Model file for the job. Use its own axes, mm. A direction names the side the tool comes from. Round coordinates to 2 decimals unless told otherwise and drop trailing zeros. Loops run counter-clockwise (first coordinate to the right, second up) from the corner with the lowest first, then second, coordinate; pieces in that order, holes last. Notation, with made-up numbers: (29.25, 12.5) -> (36.25, 12.5) arc R22 cw to (36.25, 35.5) -> close; hole circle Ø10 at (-21, 83.5). An arc over 180 degrees is marked (long way). Use a Markdown table: item, result. Add a question column.
```python
from build123d import *

# Parameters (mm, degrees)
BODY_START           = -10
BODY_DEPTH           = 20
M3_CLEARANCE_HOLE1_D = 3.4
CUT_EXTRUDE1_REACH   = 34.243
SKETCH4_R            = 2.5


# Read off the part's stored shape, not the designer's step: Body
with BuildPart() as part:
    # Body outline → Body (new body)
    with BuildSketch(Plane.XY.offset(BODY_START)):
        Polygon((9.25, 24.25), (9.25, 4.25), (-1.25, 4.25), (-1.25, 24.25), (-5.75, 24.25), (-5.75, 4.25), (-13, 4.25), (-13, -1.25), (13, -1.25), (13, 24.25), align=None)
    extrude(amount=BODY_DEPTH)

    # M3 Clearance Hole1 (through all)
    with Locations(Plane(origin=(0, -1.25, 0), x_dir=(-1, 0, 0), z_dir=(0, -1, 0))):
        with Locations((9, -3), (9, 3)):
            Hole(M3_CLEARANCE_HOLE1_D / 2)

    # Cut-Extrude1: up to this face of the body (flat: up to its plane)
    cut_extrude1_end = Plane(part.part.faces().sort_by_distance((13, 11.5, 0))[0])
    # Sketch4 → Cut-Extrude1 (cut, up to the picked face)
    with BuildSketch(Plane.ZY.offset(5.75), mode=Mode.PRIVATE) as cut_extrude1_sk1:
        with Locations((0, 14.25)):
            Circle(SKETCH4_R)
    cut_extrude1_tool1 = split(extrude(cut_extrude1_sk1.sketch, amount=-CUT_EXTRUDE1_REACH, mode=Mode.PRIVATE), bisect_by=cut_extrude1_end, keep=Keep.BOTH, mode=Mode.PRIVATE)
    add(cut_extrude1_tool1.solids().sort_by(Axis((-5.75, 14.25, 0), (1, 0, 0)))[0], mode=Mode.SUBTRACT)


solid = part.part
```
1) Tool access for faces 1 (the face through (11, 24.25, 0)), 2 (the face through (-1.25, 16, -2)), 3 (the face through (-9, 4.25, 0)): list every direction of +Z, -Z, +X, -X, +Y, -Y with a clear straight run to the whole face (end or side of a thin tool).
2) Cut at C-C on x = -9. Write the cut outline in (y, z), and give its area (3 significant figures).
3) Wall check: probe 1 along Z at (x, y) = (-9, 2.35); probe 2 along X at (y, z) = (7.75, -5.5); probe 3 along Y at (x, z) = (-4.4, 0). Give the ranges that are in metal, low to high. Write a range as from..to.
4) Cut at A-A on z = -3. Write the cut outline in (x, y).
5) Cut at D-D on z = 0. Write the cut outline in (x, y).
6) Pin check, flat tips, straight feed: pin 1 Ø10 at (x, y) = (0, 5.5) entering from +Z; pin 2 Ø6.5 at (y, z) = (14.25, 0) entering from -X; pin 3 Ø3 at (x, z) = (4.5, 2.5) entering from +Y. Stop position of each tip, or through.
7) Cut at B-B on y = 19.25. Write the cut outline in (x, z).
8) Pull direction Z, two halves, no side cores. Call faces 4 (the face through (3, 3, 10)), 5 (the face through (-13, 2, 0)), 6 (the face through (-10.25, 1.54, -4.15)): +Z half, -Z half, draft (parallel to the pull), parting line (faces both ways), or undercut.
Established:
| question | item | result |
|---|---|---|
| 1 | face 1 | +Z, -Z, +X, -X, +Y |
| 1 | face 2 | +Z, -Z, +Y |
| 1 | face 3 | +Z, -Z, -X, +Y |
| 2 | outline | (-1.25, -10) -> (4.25, -10) -> (4.25, -4.7) -> (-1.25, -4.7) -> close; (-1.25, -1.3) -> (4.25, -1.3) -> (4.25, 1.3) -> (-1.25, 1.3) -> close; (-1.25, 4.7) -> (4.25, 4.7) -> (4.25, 10) -> (-1.25, 10) -> close |
| 2 | area | 72.6 mm^2 |
| 3 | probe 1 | z = -10..-4.7, -1.3..1.3, 4.7..10 |
| 3 | probe 2 | x = -5.75..-1.25, 9.25..13 |
| 3 | probe 3 | y = -1.25..11.75, 16.75..24.25 |
| 4 | outline | (-13, -1.25) -> (-10.7, -1.25) -> (-10.7, 4.25) -> (-13, 4.25) -> close; (-7.3, -1.25) -> (13, -1.25) -> (13, 24.25) -> (9.25, 24.25) -> (9.25, 4.25) -> (-1.25, 4.25) -> (-1.25, 24.25) -> (-5.75, 24.25) -> (-5.75, 4.25) -> (-7.3, 4.25) -> close |
| 5 | outline | (-13, -1.25) -> (13, -1.25) -> (13, 11.75) -> (9.25, 11.75) -> (9.25, 4.25) -> (-1.25, 4.25) -> (-1.25, 11.75) -> (-5.75, 11.75) -> (-5.75, 4.25) -> (-13, 4.25) -> close; (-5.75, 16.75) -> (-1.25, 16.75) -> (-1.25, 24.25) -> (-5.75, 24.25) -> close; (9.25, 16.75) -> (13, 16.75) -> (13, 24.25) -> (9.25, 24.25) -> close |
| 6 | pin 1 | stops at z = 10 |
| 6 | pin 2 | stops at x = -5.75 |
| 6 | pin 3 | stops at y = 4.25 |
| 7 | outline | (-5.75, -10) -> (-1.25, -10) -> (-1.25, 10) -> (-5.75, 10) -> close; (9.25, -10) -> (13, -10) -> (13, 10) -> (9.25, 10) -> close |
| 8 | face 4 | +Z half |
| 8 | face 5 | draft |
| 8 | face 6 | undercut |
